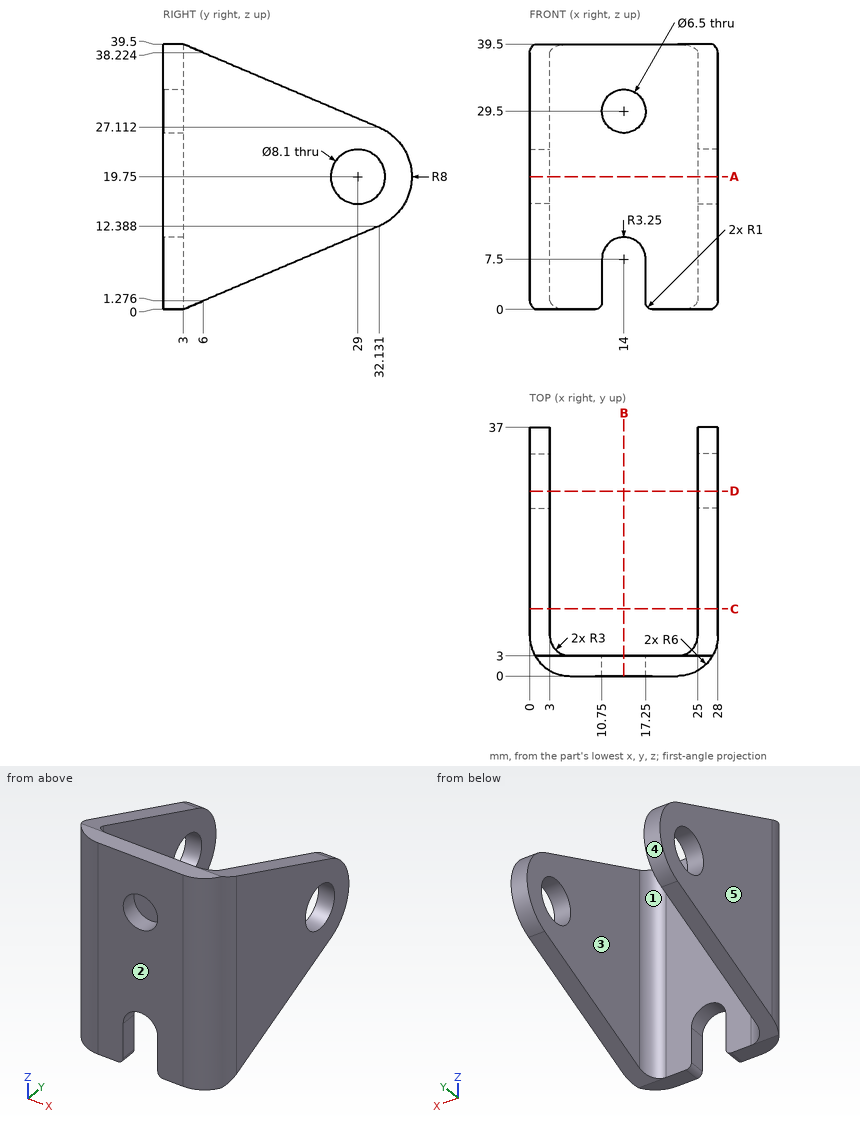
Geometry check sheet. Reference: drawing and pictorial views, mm from the part's lowest x, y, z. A direction names the side the tool comes from. Round coordinates to 2 decimals unless told otherwise and drop trailing zeros. Order: outer loops, then holes, each group sorted by start corner. A loop starts at its lowest first (then second) coordinate and runs counter-clockwise, first axis right, second up.
Q1. Set-up check for the marked faces 1 and 2: record each of +Z, -Z, +X, -X, +Y, -Y from which the full face is reachable in a straight line by a thin tool's end or side.
Filled sheet:
face 1: +Z, -Z, +Y
face 2: +Z, -Z, +X, -X, -Y
Q2. Draft check along X on the marked faces 3, 4 and 5. Enter one of: pulls with the +X half, pulls with the -X half, needs draft (parallel to the pull), parting line crosses it, or undercut.
Filled sheet:
face 3: undercut
face 4: needs draft
face 5: pulls with the -X half
Q3. Cross-section at C-C, the plane y = 10. Enter the section's corners in (x, z), plus the area to 3 significant figures.
Filled sheet:
outline: (0, 2.98) - (3, 2.98) - (3, 36.52) - (0, 36.52) - close; (25, 2.98) - (28, 2.98) - (28, 36.52) - (25, 36.52) - close
area: 201 mm2
Q4. Depth check by flat-ended pin: P1, Ø1.5, axis at y = 2, z = 6, coming from the +X side; P2, Ø10, axis at x = 15, z = 28, coming from the -Y side; P3, Ø7.5, axis at x = 14, z = 29.5, coming from the +Y side; P4, Ø2.5, axis at y = 2, z = 4.5, coming from the -X side. Enter the tip coordinate at first touch or a pass-through.
Filled sheet:
P1: stops at x = 27.04
P2: stops at y = 0
P3: stops at y = 3
P4: stops at x = 0.67
Q5. Cross-section at D-D, the plane y = 27.5. Enter the section's corners in (x, z).
Filled sheet:
outline: (0, 10.42) - (3, 10.42) - (3, 15.99) - (0, 15.99) - close; (0, 23.51) - (3, 23.51) - (3, 29.08) - (0, 29.08) - close; (25, 10.42) - (28, 10.42) - (28, 15.99) - (25, 15.99) - close; (25, 23.51) - (28, 23.51) - (28, 29.08) - (25, 29.08) - close
Q6. Cross-section at A-A, the plane z = 19.75. Enter the section's corners in (x, y).
Filled sheet:
outline: (0, 6) arc R6 ccw to (6, 0) - (22, 0) arc R6 ccw to (28, 6) - (28, 24.95) - (25, 24.95) - (25, 6) arc R3 cw to (22, 3) - (6, 3) arc R3 cw to (3, 6) - (3, 24.95) - (0, 24.95) - close; (0, 33.05) - (3, 33.05) - (3, 37) - (0, 37) - close; (25, 33.05) - (28, 33.05) - (28, 37) - (25, 37) - close
Q7. Scan lines: L1, parallel to X at y = 16, z = 18; L2, parallel to Y at x = 14.25, z = 17; L3, parallel to Y at x = 24.75, z = 14.5 (1 decimal). Record each from-to range of solid material in increasing order.
Filled sheet:
L1: x = 0 to 3, 25 to 28
L2: y = 0 to 3
L3: y = 0.7 to 4.8
Q8. Cross-section at B-B, the plane x = 14. Enter the section's corners in (y, z).
Filled sheet:
outline: (0, 10.75) - (3, 10.75) - (3, 26.25) - (0, 26.25) - close; (0, 32.75) - (3, 32.75) - (3, 39.5) - (0, 39.5) - close
